Could you check a few things on this model? Use its own coordinates, in mm. Face numbers are marked on the shaded views. A direction names the side the tool comes from. Round coordinates to 2 decimals unless told otherwise and drop trailing zeros. Loops run counter-clockwise (first coordinate to the right, second up) from the corner with the lowest first, then second, coordinate; pieces in that order, holes last. Notation, with made-up numbers: M 77,-25 L 134,-25 A13 cw 134,-13 Z; hole C -7.75,-20 d1. An arc over 180 degrees is marked long. Answer in a Markdown table with one row per item.
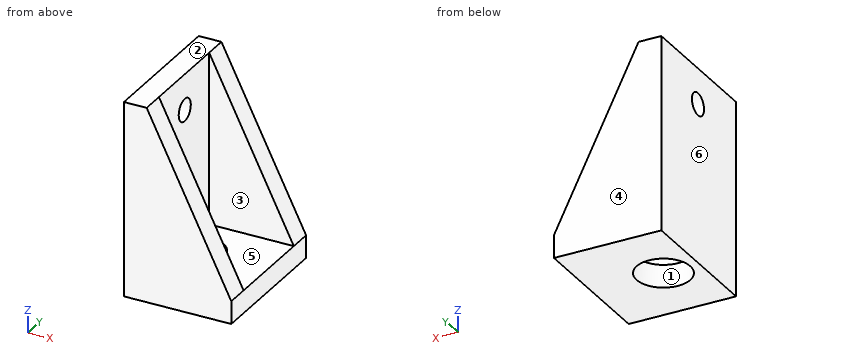
```python
from build123d import *

# Parameters (mm, degrees)
F1_DEPTH = 13
F3_DEPTH = 3.175
F5_DEPTH = 3.175
F6_R     = 3.75
F7_DEPTH = 3.176
F8_R     = 1.56
F9_DEPTH = 3.176


with BuildPart() as f1:
    # F0 (on Front) → F1 (new body)
    with BuildSketch(Plane.XZ):
        Polygon((0, 24), (-3.175, 24), (-3.175, -3.175), (11.825, -3.175), (11.825, 0), (0, 0), align=None)
    extrude(amount=F1_DEPTH)

    # F2 (on face) → F3 (join)
    with BuildSketch(Plane.XZ.offset(13)):
        Polygon((0, 24), (-3.175, 24), (-3.175, -3.175), (11.825, -3.175), (11.825, 0), align=None)
    extrude(amount=F3_DEPTH)

    # F4 (on face) → F5 (join)
    with BuildSketch(Plane(origin=(0, 0, 0), x_dir=(-1, 0, 0), z_dir=(0, 1, 0))):
        Polygon((3.175, -3.175), (3.175, 24), (0, 24), (-11.825, 0), (-11.825, -3.175), align=None)
    extrude(amount=F5_DEPTH)

    # F6 (on face) → F7 (cut, through all)
    with BuildSketch(Plane.XY):
        with Locations((1.825, -6.65)):
            Circle(F6_R)
    extrude(amount=-F7_DEPTH, mode=Mode.SUBTRACT)

    # F8 (on face) → F9 (cut, through all)
    with BuildSketch(Plane.YZ):
        with Locations((-6.313409, 19)):
            Circle(F8_R)
    extrude(amount=-F9_DEPTH, mode=Mode.SUBTRACT)


solid = f1.part
```
1) Which directions (+Z, -Z, +X, -X, +Y, -Y) give clear straight access to the entire face, cutting with the end or side of a thin tool? Please do the marked faces 5 and 6.
Computed:
| item | result |
|---|---|
| face 5 | +Z, +X |
| face 6 | +Z, -Z, -X, +Y, -Y |
2) I want a section at D-D, the plane z = 11.75. Please give me the cut outline in (x, y) (3 decimals), plus the area to 3 significant figures.
Computed:
| item | result |
|---|---|
| outline | M -3.175,-16.175 L 6.036,-16.175 L 6.036,-13 L 0,-13 L 0,0 L 6.036,0 L 6.036,3.175 L -3.175,3.175 Z |
| area | 99.8 mm² |
3) If we mould it in two halves opening along Y, with no side actions, what happens to the marked faces 1, 2, 3 and 4? For each: released by +Y, released by -Y, zero draft, split by the parting line, or undercut.
Computed:
| item | result |
|---|---|
| face 1 | undercut |
| face 2 | zero draft |
| face 3 | undercut |
| face 4 | released by +Y |
4) I want a section at B-B, the plane y = -6.65. Please give me the cut outline in (x, z) (3 decimals), plus the area to 3 significant figures.
Computed:
| item | result |
|---|---|
| outline | M -3.175,-3.175 L -1.925,-3.175 L -1.925,0 L 0,0 L 0,17.477 L -3.175,17.477 Z; M -3.175,20.523 L 0,20.523 L 0,24 L -3.175,24 Z; M 5.575,-3.175 L 11.825,-3.175 L 11.825,0 L 5.575,0 Z |
| area | 90.3 mm² |
5) I want a section at C-C, the plane y = 1. Please give me the cut outline in (x, z) (3 decimals), plus the area to 3 significant figures.
Computed:
| item | result |
|---|---|
| outline | M -3.175,-3.175 L 11.825,-3.175 L 11.825,0 L 0,24 L -3.175,24 Z |
| area | 266 mm² |
6) Will these pins go through, and if not, where does the flat tip stop? P1, Ø4, axis at x = 5, y = -8.5, coming from the +Z side; P2, Ø4, axis at y = -3.5, z = 17, coming from the +X side.
Computed:
| item | result |
|---|---|
| P1 | stops at z = 0 |
| P2 | stops at x = 0 |
7) I want a section at A-A, the plane z = 19. Please give me the cut outline in (x, y) (3 decimals), plus the area to 3 significant figures.
Computed:
| item | result |
|---|---|
| outline | M -3.175,-16.175 L 2.464,-16.175 L 2.464,-13 L 0,-13 L 0,-7.873 L -3.175,-7.873 Z; M -3.175,-4.753 L 0,-4.753 L 0,0 L 2.464,0 L 2.464,3.175 L -3.175,3.175 Z |
| area | 67.2 mm² |
8) I need wall thicknesses on line 1 (Y direction, x = 6, z = 6.25) (3 decimals); line 2 (X direction, y = -6.65, z = -1.6) (3 decimals); line 3 (X direction, y = -3.5, z = 9) (3 decimals). Which ranges of each line are inside material? Lowest first, please.
Computed:
| item | result |
|---|---|
| line 1 | y = -16.175 to -13, 0 to 3.175 |
| line 2 | x = -3.175 to -1.925, 5.575 to 11.825 |
| line 3 | x = -3.175 to 0 |
